Read the model definition and answer for the solid it produces. Units are mm, in the model's axes. Face numbers are marked on the shaded views. A direction names the side the tool comes from. Coordinates: 2 decimals unless noted, no trailing zeros. Loops run counter-clockwise (first coordinate to the right, second up) from the corner with the lowest first, then second, coordinate; pieces in that order, holes last. Notation, with made-up numbers: (45.5, -39.5) - (84.5, -39.5) arc R13 cw to (84.5, -34.5) - close; hole circle Ø1 at (7.5, 0). An arc over 180 degrees is marked (long way). Use one line per item in the form item = value. Start each with the question number.
1) Each of these flat-tipped pins is pushed along its axis until it touches: P1, Ø10, axis at x = 25.4, y = 708.58, coming from the +Z side; P2, Ø10, axis at x = 61.5, y = 653.5, coming from the +Z side; P3, Ø1, axis at y = 622.5, z = 614, coming from the -X side. Where does it stop, or does it pass through?
2) A cutting plane is placed at A-A (x = 13). Give the vertices of the cut face in (y, z), and give its area (3 significant figures).
3) Consider line 1 (Z direction, x = 5.5, y = 587.5); line 2 (X direction, y = 708.5, z = 740); line 3 (Z direction, x = 40, y = 718). Determine where each line is inside the solid, lowest interval first.
4) Which of the six approach directions +Z, -Z, +X, -X, +Y, -Y give full straight-line access (tool end or side, diameter ignored) to the marked faces 1 and 2?
5) A cutting plane is placed at C-C (z = 753.5). Give the vertices of the cut face in (x, y).
6) A cutting plane is placed at B-B (y = 659). Give the vertices of the cut face in (x, z), and give its area (3 significant figures).
7) The mould has two halves that part along Z. Classify the marked faces 3, 4 and 5: released by +Z, released by -Z, zero draft, split by the parting line, or undercut.
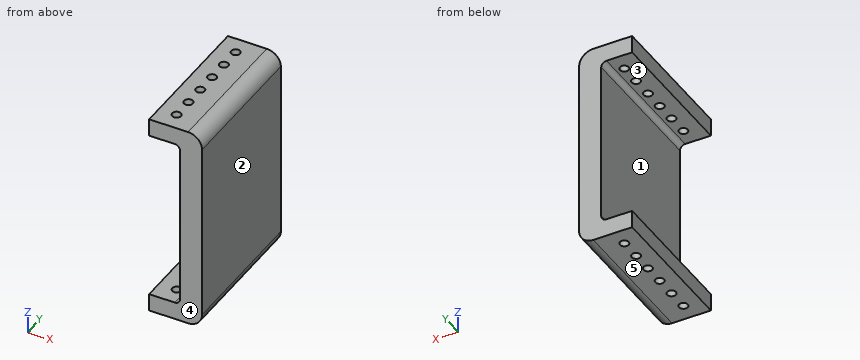
from build123d import *

# Parameters (mm, degrees)
SKETCH1_W           = 297.434
SKETCH1_H           = 203.2
BOSS_EXTRUDE1_DEPTH = 76.2
SKETCH3_W           = 44.45
SKETCH3_H           = 246.634
CUT_EXTRUDE1_DEPTH  = 204.2
SKETCH4_R           = 6.35
CUT_EXTRUDE2_DEPTH  = 298.434
FILLET1_R           = 20.32
FILLET2_R           = 7.62


with BuildPart() as part:
    # Sketch1 → Boss-Extrude1 (new body)
    with BuildSketch(Plane(origin=(0, 0, 0), x_dir=(0, 0, -1), z_dir=(1, 0, 0))):
        with Locations((-688.794526316, 662.857561404)):
            Rectangle(SKETCH1_W, SKETCH1_H)
    extrude(amount=BOSS_EXTRUDE1_DEPTH)

    # Sketch3 → Cut-Extrude1 (cut, through all)
    with BuildSketch(Plane(origin=(0, 764.457561404, 0), x_dir=(1, 0, 0), z_dir=(0, 1, 0))):
        with Locations((22.225, -688.794526316)):
            Rectangle(SKETCH3_W, SKETCH3_H)
    extrude(amount=-CUT_EXTRUDE1_DEPTH, mode=Mode.SUBTRACT)

    # Sketch4 → Cut-Extrude2 (cut, through all)
    with BuildSketch(Plane.XY.offset(837.511526316)):
        with Locations((25.4, 739.057561404)):
            Circle(SKETCH4_R)
        with Locations((25.4, 708.577561404)):
            Circle(SKETCH4_R)
        with Locations((25.4, 678.097561404)):
            Circle(SKETCH4_R)
        with Locations((25.4, 647.617561404)):
            Circle(SKETCH4_R)
        with Locations((25.4, 617.137561404)):
            Circle(SKETCH4_R)
        with Locations((25.4, 586.657561404)):
            Circle(SKETCH4_R)
    extrude(amount=-CUT_EXTRUDE2_DEPTH, mode=Mode.SUBTRACT)

    # Fillet1
    fillet1_edges = [part.edges().sort_by_distance(p)[0] for p in [
        (76.2, 662.857561404, 540.077526316),
        (76.2, 662.857561404, 837.511526316),
    ]]
    fillet(fillet1_edges, radius=FILLET1_R)

    # Fillet2
    fillet2_edges = [part.edges().sort_by_distance(p)[0] for p in [
        (44.45, 662.857561404, 565.477526316),
        (44.45, 662.857561404, 812.111526316),
    ]]
    fillet(fillet2_edges, radius=FILLET2_R)


solid = part.part
Found:
q1.P1 = through
q1.P2 = 837.5
q1.P3 = 44.45
q2.outline = (561.26, 540.08) - (764.46, 540.08) - (764.46, 565.48) - (561.26, 565.48) - close; (561.26, 812.11) - (764.46, 812.11) - (764.46, 837.51) - (561.26, 837.51) - close
q2.area = 10,300 mm^2
q3.line_1 = 540.08 to 565.48, 812.11 to 837.51
q3.line_2 = 44.45 to 76.2
q3.line_3 = 540.08 to 566.17, 811.42 to 837.51
q4.face_1 = -X, +Y, -Y
q4.face_2 = +Z, -Z, +X, +Y, -Y
q5.outline = (44.45, 561.26) - (76.2, 561.26) - (76.2, 764.46) - (44.45, 764.46) - close
q6.outline = (0, 540.08) - (55.88, 540.08) arc R20.32 ccw to (76.2, 560.4) - (76.2, 817.19) arc R20.32 ccw to (55.88, 837.51) - (0, 837.51) - (0, 812.11) - (36.83, 812.11) arc R7.62 cw to (44.45, 804.49) - (44.45, 573.1) arc R7.62 cw to (36.83, 565.48) - (0, 565.48) - close
q6.area = 11,500 mm^2
q7.face_3 = undercut
q7.face_4 = zero draft
q7.face_5 = released by -Z
